Model file for the job. Use its own axes, mm. Round coordinates to 2 decimals unless told otherwise and drop trailing zeros. Order: outer loops, then holes, each group sorted by start corner. A loop starts at its lowest first (then second) coordinate and runs counter-clockwise, first axis right, second up. Notation, with made-up numbers: (48, -17) -> (89, -17) arc R24 cw to (89, 1) -> close; hole circle Ø11 at (12, 7). An arc over 180 degrees is marked (long way). Answer as CSV lines item,"result".
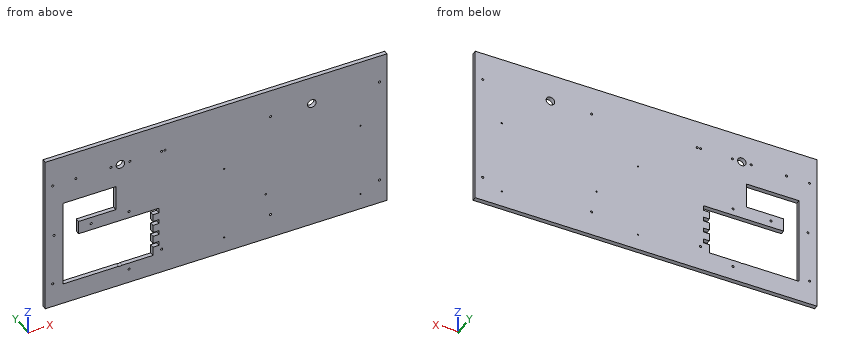
```python
from build123d import *

# Parameters (mm, degrees)
SKETCH2_W           = 400
SKETCH2_H           = 190.8
BOSS_EXTRUDE1_DEPTH = 5
SKETCH3_R           = 5
CUT_EXTRUDE1_DEPTH  = 223.556172685
SKETCH4_R           = 1.25
CUT_EXTRUDE2_DEPTH  = 223.556172685
CUT_EXTRUDE3_DEPTH  = 223.556172685
SKETCH7_R           = 0.75
CUT_EXTRUDE4_DEPTH  = 223.556172685
SKETCH8_R           = 1.25
CUT_EXTRUDE5_DEPTH  = 10
SKETCH9_R           = 1.25
CUT_EXTRUDE6_DEPTH  = 223.556172685


with BuildPart() as part:
    # Sketch2 → Boss-Extrude1 (new body)
    with BuildSketch(Plane(origin=(0, 0, 0), x_dir=(1, 0, 0), z_dir=(0, 1, 0))):
        with Locations((0, -2.1)):
            Rectangle(SKETCH2_W, SKETCH2_H)
    extrude(amount=BOSS_EXTRUDE1_DEPTH)

    # Sketch3 → Cut-Extrude1 (cut, through all)
    with BuildSketch(Plane(origin=(0, 5, 0), x_dir=(1, 0, 0), z_dir=(0, 1, 0))):
        with Locations(Location((-112, 63.75, 0), (0, 0, 270))):
            Circle(SKETCH3_R)
        with Locations(Location((112, -63.75, 0), (0, 0, 270))):
            Circle(SKETCH3_R)
        with Locations(Location((-112, -63.75, 0), (0, 0, 270))):
            Circle(SKETCH3_R)
    extrude(amount=-CUT_EXTRUDE1_DEPTH, mode=Mode.SUBTRACT)

    # Sketch4 → Cut-Extrude2 (cut, through all)
    with BuildSketch(Plane(origin=(0, 5, 0), x_dir=(1, 0, 0), z_dir=(0, 1, 0))):
        with Locations(Location((-191.25, 63.75, 0), (0, 0, 270))):
            Circle(SKETCH4_R)
        with Locations(Location((-63.75, 63.75, 0), (0, 0, 270))):
            Circle(SKETCH4_R)
        with Locations(Location((63.75, 63.75, 0), (0, 0, 270))):
            Circle(SKETCH4_R)
        with Locations(Location((191.25, 63.75, 0), (0, 0, 270))):
            Circle(SKETCH4_R)
        with Locations(Location((191.25, -63.75, 0), (0, 0, 270))):
            Circle(SKETCH4_R)
        with Locations(Location((63.75, -63.75, 0), (0, 0, 270))):
            Circle(SKETCH4_R)
        with Locations(Location((-63.75, -63.75, 0), (0, 0, 270))):
            Circle(SKETCH4_R)
        with Locations(Location((-191.25, -63.75, 0), (0, 0, 270))):
            Circle(SKETCH4_R)
    extrude(amount=-CUT_EXTRUDE2_DEPTH, mode=Mode.SUBTRACT)

    # Sketch5 → Cut-Extrude3 (cut, through all)
    with BuildSketch(Plane(origin=(0, 5, 0), x_dir=(1, 0, 0), z_dir=(0, 1, 0))):
        Polygon((-179, 68.3), (-179, -36.7), (-117.327189105, -36.7), (-117.327189105, -6.7), (-161, -6.7), (-161, 9.3), (-67, 9.3), (-67, 15.3), (-74, 15.3), (-74, 24.252605128), (-67, 24.252605128), (-67, 29.252605128), (-74, 29.252605128), (-74, 38.451162805), (-67, 38.451162805), (-67, 43.451162805), (-74, 43.451162805), (-74, 52.70528249), (-67, 52.70528249), (-67, 57.70528249), (-74, 57.70528249), (-74, 68.3), (-76.383096774, 68.3), align=None)
    extrude(amount=-CUT_EXTRUDE3_DEPTH, mode=Mode.SUBTRACT)

    # Sketch7 → Cut-Extrude4 (cut, through all)
    with BuildSketch(Plane(origin=(0, 5, 0), x_dir=(1, 0, 0), z_dir=(0, 1, 0))):
        with Locations(Location((9.399984, 74.29999922, 0), (0, 0, 270))):
            Circle(SKETCH7_R)
        with Locations(Location((58.062496917, 35.300001471, 0), (0, 0, 270))):
            Circle(SKETCH7_R)
        with Locations(Location((168.9, 74.29999922, 0), (0, 0, 270))):
            Circle(SKETCH7_R)
        with Locations(Location((168.9, -14.70000278, 0), (0, 0, 270))):
            Circle(SKETCH7_R)
        with Locations(Location((9.399984, -14.70000278, 0), (0, 0, 270))):
            Circle(SKETCH7_R)
    extrude(amount=-CUT_EXTRUDE4_DEPTH, mode=Mode.SUBTRACT)

    # Sketch8 → Cut-Extrude5 (cut)
    with BuildSketch(Plane(origin=(0, 5, 0), x_dir=(1, 0, 0), z_dir=(0, 1, 0))):
        with Locations(Location((-164.2, -63.75, 0), (0, 0, 270))):
            Circle(SKETCH8_R)
        with Locations(Location((-123, -63.75, 0), (0, 0, 270))):
            Circle(SKETCH8_R)
        with Locations(Location((-101, -63.75, 0), (0, 0, 270))):
            Circle(SKETCH8_R)
        with Locations(Location((-59.8, -63.75, 0), (0, 0, 270))):
            Circle(SKETCH8_R)
    extrude(amount=-CUT_EXTRUDE5_DEPTH, mode=Mode.SUBTRACT)

    # Sketch9 → Cut-Extrude6 (cut, through all)
    with BuildSketch(Plane(origin=(0, 5, 0), x_dir=(1, 0, 0), z_dir=(0, 1, 0))):
        with Locations(Location((-189.5, 1.3, 0), (0, 0, 270))):
            Circle(SKETCH9_R)
        with Locations(Location((-146.206430225, 1.3, 0), (0, 0, 270))):
            Circle(SKETCH9_R)
        with Locations(Location((-101.86, 76.3, 0), (0, 0, 270))):
            Circle(SKETCH9_R)
        with Locations(Location((-101.86, 1.3, 0), (0, 0, 270))):
            Circle(SKETCH9_R)
    extrude(amount=-CUT_EXTRUDE6_DEPTH, mode=Mode.SUBTRACT)


solid = part.part
```
Q1. Saw through at B-B (x = -140). Write the cut outline in (y, z).
Checks:
outline,"(0, -93.3) -> (5, -93.3) -> (5, -68.3) -> (0, -68.3) -> close; (0, -9.3) -> (5, -9.3) -> (5, 6.7) -> (0, 6.7) -> close; (0, 36.7) -> (5, 36.7) -> (5, 97.5) -> (0, 97.5) -> close"
Q2. Saw through at D-D (y = 2.7). State how many separate pieces and enclosed holes the cut face has, plus the area to 3 significant figures.
Checks:
separate pieces,"1"
enclosed holes,"24"
area,"67,600 mm²"
Q3. Wall check: L1, parallel to X at y = 0.3, z = -74; L2, parallel to X at y = 1.45, z = -63.75; L3, parallel to Z at x = -60, y = 2.4. Give the ranges that are in metal, low to high. Write a range as [from, to].
Checks:
L1,"[-200, 8.71], [10.09, 168.21], [169.59, 200]"
L2,"[-200, -192.5], [-190, -179], [-74, -65], [-62.5, 62.5], [65, 190], [192.5, 200]"
L3,"[-93.3, 62.52], [64.98, 97.5]"
Q4. Flat gauge pin, fed straight in: pin 1 (2 mm diameter, centred on x = -191.25, z = 63.75, fed in from -Y). Where does the tip first touch, or does it go through?
Checks:
pin 1,"through"
Q5. Saw through at A-A (x = 112). Write the cut outline in (y, z), plus the area to 3 significant figures.
Checks:
outline,"(0, -93.3) -> (5, -93.3) -> (5, 58.75) -> (0, 58.75) -> close; (0, 68.75) -> (5, 68.75) -> (5, 97.5) -> (0, 97.5) -> close"
area,"904 mm²"
Q6. Saw through at C-C (x = -92). Write the cut outline in (y, z), plus the area to 3 significant figures.
Checks:
outline,"(0, -93.3) -> (5, -93.3) -> (5, -68.3) -> (0, -68.3) -> close; (0, -9.3) -> (5, -9.3) -> (5, 97.5) -> (0, 97.5) -> close"
area,"659 mm²"
